from build123d import *

# Parameters (mm, degrees)
F2_DEPTH        = 2.5
F2_COPIES_COUNT = 11
F3_DEPTH        = 2.5


# Not quite as in the source:
# - a pattern or mirror of a feature is missing from the dataset's text; its kind, count and spacing are read off the source's solid


with BuildPart() as f2:
    # F1 (on Front) → F2 (new body)
    with BuildSketch(Plane.XZ):
        with BuildLine():
            ThreePointArc((1.9034310201, 12.7798019983), (1.2593174989, 14.5936400637), (0.2749085502, 16.2476744579))
            ThreePointArc((0.2749085502, 16.2476744579), (0, 16.25), (-0.2749085502, 16.2476744579))
            ThreePointArc((-0.2749085502, 16.2476744579), (-1.2593174989, 14.5936400637), (-1.9034310201, 12.7798019983))
            Line((-1.9034310201, 12.7798019983), (-1.5652278506, 10.5090763998))
            ThreePointArc((-1.5652278506, 10.5090763998), (0, 10.625), (1.5652278506, 10.5090763998))
            Line((1.5652278506, 10.5090763998), (1.9034310201, 12.7798019983))
        make_face()
    extrude(amount=F2_DEPTH)


with BuildPart() as f2_copies_1:
    # F2_copies: instance of F2
    add(f2.part.rotate(Axis((0, 0, 0), (0, 1, 0)), 1 * 360 / F2_COPIES_COUNT))


with BuildPart() as f2_copies_2:
    # F2_copies: instance of F2
    add(f2.part.rotate(Axis((0, 0, 0), (0, 1, 0)), 2 * 360 / F2_COPIES_COUNT))


with BuildPart() as f2_copies_3:
    # F2_copies: instance of F2
    add(f2.part.rotate(Axis((0, 0, 0), (0, 1, 0)), 3 * 360 / F2_COPIES_COUNT))


with BuildPart() as f2_copies_4:
    # F2_copies: instance of F2
    add(f2.part.rotate(Axis((0, 0, 0), (0, 1, 0)), 4 * 360 / F2_COPIES_COUNT))


with BuildPart() as f2_copies_5:
    # F2_copies: instance of F2
    add(f2.part.rotate(Axis((0, 0, 0), (0, 1, 0)), 5 * 360 / F2_COPIES_COUNT))


with BuildPart() as f2_copies_6:
    # F2_copies: instance of F2
    add(f2.part.rotate(Axis((0, 0, 0), (0, 1, 0)), 6 * 360 / F2_COPIES_COUNT))


with BuildPart() as f2_copies_7:
    # F2_copies: instance of F2
    add(f2.part.rotate(Axis((0, 0, 0), (0, 1, 0)), 7 * 360 / F2_COPIES_COUNT))


with BuildPart() as f2_copies_8:
    # F2_copies: instance of F2
    add(f2.part.rotate(Axis((0, 0, 0), (0, 1, 0)), 8 * 360 / F2_COPIES_COUNT))


with BuildPart() as f2_copies_9:
    # F2_copies: instance of F2
    add(f2.part.rotate(Axis((0, 0, 0), (0, 1, 0)), 9 * 360 / F2_COPIES_COUNT))


with BuildPart() as f2_copies_10:
    # F2_copies: instance of F2
    add(f2.part.rotate(Axis((0, 0, 0), (0, 1, 0)), 10 * 360 / F2_COPIES_COUNT))


with BuildPart() as f2_1:
    add(f2.part)

    add(f2_copies_1.part)  # F3 merges F2_copies_1

    add(f2_copies_2.part)  # F3 merges F2_copies_2

    add(f2_copies_3.part)  # F3 merges F2_copies_3

    add(f2_copies_4.part)  # F3 merges F2_copies_4

    add(f2_copies_5.part)  # F3 merges F2_copies_5

    add(f2_copies_6.part)  # F3 merges F2_copies_6

    add(f2_copies_7.part)  # F3 merges F2_copies_7

    add(f2_copies_8.part)  # F3 merges F2_copies_8

    add(f2_copies_9.part)  # F3 merges F2_copies_9

    add(f2_copies_10.part)  # F3 merges F2_copies_10
    # F1 (on Front) → F3 (join)
    with BuildSketch(Plane.XZ):
        with BuildLine():
            ThreePointArc((10.625, 0), (8.0473961911, 6.9375816784), (1.5652278506, 10.5090763998))
            ThreePointArc((1.5652278506, 10.5090763998), (0, 10.625), (-1.5652278506, 10.5090763998))
            ThreePointArc((-1.5652278506, 10.5090763998), (-6.9375816784, -8.0473961911), (10.625, 0))
        make_face()
    extrude(amount=F3_DEPTH)


solid = f2_1.part
Geometry check sheet. Reference: the model listing, model coordinates, mm. A direction names the side the tool comes from. Give positions to 0.01 mm unless a question says otherwise; leave off trailing zeros. Order: outer loops, then holes, each group sorted by start corner. A loop starts at its lowest first (then second) coordinate and runs counter-clockwise, first axis right, second up.
1. Draft check along Z on faces 5 (the face through (12.779, -1.232, 7.208)), 6 (the face through (-8.02, -1.23, 6.97)), 7 (the face through (10.18, -1.23, -10.5)). Enter one of: pulls with the +Z half, pulls with the -Z half, needs draft (parallel to the pull), parting line crosses it, or undercut.
Completed:
face 5: pulls with the +Z half
face 6: undercut
face 7: pulls with the -Z half
2. Access from +Z, -Z, +X, -X, +Y, -Y to the whole of each face (thin tool, end or side, straight path). Record for faces 1 (the face through (9.95, -1.232, -6.323)), 2 (the face through (-1.737, -1.232, 11.66)), 3 (the face through (6.9, -1.2, 13)), 4 (the face through (-7.765, -1.232, 8.87)).
Completed:
face 1: +X, +Y, -Y
face 2: +Y, -Y
face 3: +Z, +Y, -Y
face 4: -X, +Y, -Y
3. Sectioned sample at D-D (z = 0.5). Record the boundary of the cut face in (x, y).
Completed:
outline: (-10.61, -2.5) - (10.61, -2.5) - (10.61, 0) - (-10.61, 0) - close
4. Sectioned sample at A-A (x = -11.5). Record the boundary of the cut face in (y, z), then the cut area to 3 significant figures.
Completed:
outline: (-2.5, -10.78) - (0, -10.78) - (0, -7.89) - (-2.5, -7.89) - close; (-2.5, -3.44) - (0, -3.44) - (0, 0.06) - (-2.5, 0.06) - close; (-2.5, 3.31) - (0, 3.31) - (0, 7.14) - (-2.5, 7.14) - close
area: 25.5 mm2
5. Sectioned sample at C-C (x = 3.5). Record the boundary of the cut face in (y, z).
Completed:
outline: (-2.5, -14.97) - (0, -14.97) - (0, 10.03) - (-2.5, 10.03) - close
6. Scan lines: line 1 (Z direction, x = -11.5, y = -2.2); line 2 (X direction, y = -1.5, z = 13.5); line 3 (Z direction, x = -8, y = -1.9). Record each from-to range of solid material in increasing order.
Completed:
line 1: z = -10.78 to -7.89, -3.44 to 0.06, 3.31 to 7.14
line 2: x = -9.02 to -7.81, -1.7 to 1.7, 7.81 to 9.02
line 3: z = -9.33 to 6.99, 9.14 to 13.59
7. Depth check by flat-ended pin: pin 1 (4 mm diameter, centred on x = -6, z = 3, fed in from +Y); pin 2 (2 mm diameter, centred on x = 3, z = 12, fed in from -Y); pin 3 (1.5 mm diameter, centred on y = -1, z = 7, fed in from +X). Enter the tip coordinate at first touch or a pass-through.
Completed:
pin 1: stops at y = 0
pin 2: passes through
pin 3: stops at x = 14.89
8. Sectioned sample at B-B (z = -9). Record the boundary of the cut face in (x, y), then the cut area to 3 significant figures.
Completed:
outline: (-12.02, -2.5) - (-7.72, -2.5) - (-7.72, 0) - (-12.02, 0) - close; (-5.65, -2.5) - (5.65, -2.5) - (5.65, 0) - (-5.65, 0) - close; (7.72, -2.5) - (12.02, -2.5) - (12.02, 0) - (7.72, 0) - close
area: 49.7 mm2
